Model file for the job. Use its own axes, mm. Face numbers are marked on the shaded views. A direction names the side the tool comes from. Round coordinates to 2 decimals unless told otherwise and drop trailing zeros. Order: outer loops, then holes, each group sorted by start corner. A loop starts at its lowest first (then second) coordinate and runs counter-clockwise, first axis right, second up. Notation, with made-up numbers: (48, 77.25) -> (83, 77.25) arc R22 cw to (83, 114.25) -> close; hole circle Ø11 at (-9.5, 26). An arc over 180 degrees is marked (long way). Answer as CSV lines item,"result".
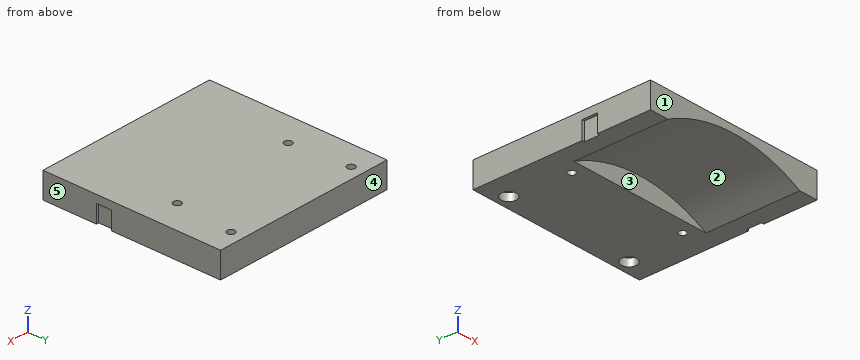
```python
from build123d import *

# Parameters (mm, degrees)
BOX241_W           = 6
BOX241_H           = 6
BOX241_DEPTH       = 64
BOX240_W           = 6
BOX240_H           = 6
BOX240_DEPTH       = 64
CYLINDER_R         = 60.2
CYLINDER_DEPTH     = 52
CYLINDER1233_R     = 1.5
CYLINDER1233_DEPTH = 32
CYLINDER1232_R     = 1.5
CYLINDER1232_DEPTH = 32
CYLINDER1239_R     = 1.5
CYLINDER1239_DEPTH = 100
CYLINDER1238_R     = 1.5
CYLINDER1238_DEPTH = 100
CYLINDER1245_R     = 3
CYLINDER1245_DEPTH = 3
CYLINDER1244_R     = 3
CYLINDER1244_DEPTH = 3
CYLINDER544_R      = 1.5
CYLINDER544_DEPTH  = 50
CYLINDER550_R      = 1.5
CYLINDER550_DEPTH  = 50
CYLINDER556_R      = 1.5
CYLINDER556_DEPTH  = 50
CYLINDER549_R      = 1.5
CYLINDER549_DEPTH  = 50
CYLINDER535_R      = 1.5
CYLINDER535_DEPTH  = 100
CYLINDER538_R      = 1.5
CYLINDER538_DEPTH  = 100
CYLINDER583_R      = 1.5
CYLINDER583_DEPTH  = 100
CYLINDER584_R      = 1.5
CYLINDER584_DEPTH  = 100
BOX142_W           = 72
BOX142_H           = 70
BOX142_DEPTH       = 10


with BuildPart() as krychle241:
    # Box241 → Box241 (new body)
    with BuildSketch(Plane(origin=(87, -3, -93), x_dir=(1, 0, 0), z_dir=(0, 0, 1))):
        with Locations((3, 3)):
            Rectangle(BOX241_W, BOX241_H)
    extrude(amount=BOX241_DEPTH)


with BuildPart() as compound653:
    # Box240 → Box240 (new body)
    with BuildSketch(Plane(origin=(11, -3, -93), x_dir=(1, 0, 0), z_dir=(0, 0, 1))):
        with Locations((3, 3)):
            Rectangle(BOX240_W, BOX240_H)
    extrude(amount=BOX240_DEPTH)

    # Compound653: union Krychle241
    add(krychle241.part)


with BuildPart() as compound653_1:
    # Compound653 placement: moved
    add(compound653.part.moved(Location((-52, 0, 36))))


with BuildPart() as obj1:
    # Cylinder → Cylinder (new body)
    with BuildSketch(Plane(origin=(0, 13, -53), x_dir=(1, 0, 0), z_dir=(0, -1, 0))):
        Circle(CYLINDER_R)
    extrude(amount=CYLINDER_DEPTH)


with BuildPart() as obj2:
    # Cylinder1233 → Cylinder1233 (new body)
    with BuildSketch(Plane(origin=(78, 41, -42), x_dir=(1, 0, 0), z_dir=(0, 0, 1))):
        Circle(CYLINDER1233_R)
    extrude(amount=CYLINDER1233_DEPTH)


with BuildPart() as compound620:
    # Cylinder1232 → Cylinder1232 (new body)
    with BuildSketch(Plane(origin=(26, 41, -42), x_dir=(1, 0, 0), z_dir=(0, 0, 1))):
        Circle(CYLINDER1232_R)
    extrude(amount=CYLINDER1232_DEPTH)

    # Compound620: union obj2
    add(obj2.part)


with BuildPart() as compound620_1:
    # Compound620 placement: moved
    add(compound620.part.moved(Location((-52, 0, 36))))


with BuildPart() as obj3:
    # Cylinder1239 → Cylinder1239 (new body)
    with BuildSketch(Plane(origin=(14, 0, -60), x_dir=(1, 0, 0), z_dir=(0, 0, 1))):
        Circle(CYLINDER1239_R)
    extrude(amount=CYLINDER1239_DEPTH)


with BuildPart() as compound630:
    # Cylinder1238 → Cylinder1238 (new body)
    with BuildSketch(Plane(origin=(90, 0, -60), x_dir=(1, 0, 0), z_dir=(0, 0, 1))):
        Circle(CYLINDER1238_R)
    extrude(amount=CYLINDER1238_DEPTH)

    # Compound625: union obj3
    add(obj3.part)


with BuildPart() as compound630_1:
    # Compound625 placement: moved
    add(compound630.part.moved(Location((-52, 0, 0))))

    # Compound630: union Compound620
    add(compound620_1.part)


with BuildPart() as obj4:
    # Cylinder1245 → Cylinder1245 (new body)
    with BuildSketch(Plane(origin=(78, 41, -42), x_dir=(1, 0, 0), z_dir=(0, 0, 1))):
        Circle(CYLINDER1245_R)
    extrude(amount=CYLINDER1245_DEPTH)


with BuildPart() as compound634:
    # Cylinder1244 → Cylinder1244 (new body)
    with BuildSketch(Plane(origin=(26, 41, -42), x_dir=(1, 0, 0), z_dir=(0, 0, 1))):
        Circle(CYLINDER1244_R)
    extrude(amount=CYLINDER1244_DEPTH)

    # Compound634: union obj4
    add(obj4.part)


with BuildPart() as compound634_1:
    # Compound634 placement: moved
    add(compound634.part.moved(Location((-52, 0, 42))))


with BuildPart() as obj5:
    # Cylinder544 → Cylinder544 (new body)
    with BuildSketch(Plane(origin=(-51, 6, 0), x_dir=(1, 0, 0), z_dir=(0, 0, 1))):
        Circle(CYLINDER544_R)
    extrude(amount=CYLINDER544_DEPTH)


with BuildPart() as obj6:
    # Cylinder550 → Cylinder550 (new body)
    with BuildSketch(Plane(origin=(-24, 18, 0), x_dir=(1, 0, 0), z_dir=(0, 0, 1))):
        Circle(CYLINDER550_R)
    extrude(amount=CYLINDER550_DEPTH)


with BuildPart() as obj7:
    # Cylinder556 → Cylinder556 (new body)
    with BuildSketch(Plane(origin=(24, 18, 0), x_dir=(1, 0, 0), z_dir=(0, 0, 1))):
        Circle(CYLINDER556_R)
    extrude(amount=CYLINDER556_DEPTH)


with BuildPart() as compound324:
    # Cylinder549 → Cylinder549 (new body)
    with BuildSketch(Plane(origin=(51, 6, 0), x_dir=(1, 0, 0), z_dir=(0, 0, 1))):
        Circle(CYLINDER549_R)
    extrude(amount=CYLINDER549_DEPTH)

    # Compound324: union obj5, obj6, obj7
    add(obj5.part)
    add(obj6.part)
    add(obj7.part)


with BuildPart() as obj8:
    # Cylinder535 → Cylinder535 (new body)
    with BuildSketch(Plane(origin=(51, -12, 0), x_dir=(1, 0, 0), z_dir=(0, 0, 1))):
        Circle(CYLINDER535_R)
    extrude(amount=CYLINDER535_DEPTH)


with BuildPart() as compound323:
    # Cylinder538 → Cylinder538 (new body)
    with BuildSketch(Plane(origin=(-51, -12, 0), x_dir=(1, 0, 0), z_dir=(0, 0, 1))):
        Circle(CYLINDER538_R)
    extrude(amount=CYLINDER538_DEPTH)

    # Compound323: union obj8
    add(obj8.part)


with BuildPart() as obj9:
    # Cylinder583 → Cylinder583 (new body)
    with BuildSketch(Plane(origin=(39, -21, 0), x_dir=(1, 0, 0), z_dir=(0, 0, 1))):
        Circle(CYLINDER583_R)
    extrude(amount=CYLINDER583_DEPTH)


with BuildPart() as compound628:
    # Cylinder584 → Cylinder584 (new body)
    with BuildSketch(Plane(origin=(-39, -21, 0), x_dir=(1, 0, 0), z_dir=(0, 0, 1))):
        Circle(CYLINDER584_R)
    extrude(amount=CYLINDER584_DEPTH)

    # Compound339: union obj9
    add(obj9.part)

    # Compound628: union Compound324, Compound323
    add(compound324.part)
    add(compound323.part)


with BuildPart() as compound628_1:
    # Compound628 placement: moved
    add(compound628.part.moved(Location((0, 0, -10))))


with BuildPart() as cut209:
    # Box142 → Box142 (new body)
    with BuildSketch(Plane(origin=(-36, -24, 0), x_dir=(1, 0, 0), z_dir=(0, 0, 1))):
        with Locations((36, 35)):
            Rectangle(BOX142_W, BOX142_H)
    extrude(amount=BOX142_DEPTH)

    # Cut201: cut Compound628
    add(compound628_1.part, mode=Mode.SUBTRACT)

    # Cut202: cut Compound634
    add(compound634_1.part, mode=Mode.SUBTRACT)

    # Cut203: cut Compound630
    add(compound630_1.part, mode=Mode.SUBTRACT)

    # Cut208: cut obj1
    add(obj1.part, mode=Mode.SUBTRACT)

    # Cut209: cut Compound653
    add(compound653_1.part, mode=Mode.SUBTRACT)


solid = cut209.part
```
Q1. Saw through at C-C (x = 4). Write the cut outline in (y, z), plus the area to 3 significant figures.
Checks:
outline,"(-24, 7.07) -> (13, 7.07) -> (13, 0) -> (46, 0) -> (46, 10) -> (-24, 10) -> close"
area,"439 mm²"
Q2. Flat gauge pins, fed straight in: pin 1 (0.8 mm diameter, centred on x = -35.5, y = 0.5, fed in from -Z); pin 2 (3 mm diameter, centred on y = -1, z = 4.5, fed in from -X); pin 3 (3 mm diameter, centred on x = -25, y = 40.5, fed in from -Z). Where does each tip first touch, or does it go through?
Checks:
pin 1,"z = 7"
pin 2,"x = -35"
pin 3,"z = 3"
Q3. Saw through at B-B (z = 5.25). Write the cut outline in (x, y).
Checks:
outline,"(-36, -24) -> (-15.2, -24) -> (-15.2, 13) -> (15.2, 13) -> (15.2, -24) -> (36, -24) -> (36, -3) -> (35, -3) -> (35, 3) -> (36, 3) -> (36, 46) -> (-36, 46) -> (-36, 3) -> (-35, 3) -> (-35, -3) -> (-36, -3) -> close; hole circle Ø3 at (-26, 41); hole circle Ø3 at (-24, 18); hole circle Ø3 at (24, 18); hole circle Ø3 at (26, 41)"
Q4. Wall check: L1, parallel to X at y = 18, z = 6; L2, parallel to X at y = 41, z = 5.75; L3, parallel to Y at x = 24, z = 5. Give the ranges that are in metal, low to high. Write a range as [from, to].
Checks:
L1,"[-36, -25.5], [-22.5, 22.5], [25.5, 36]"
L2,"[-36, -27.5], [-24.5, 24.5], [27.5, 36]"
L3,"[-24, 16.5], [19.5, 46]"
Q5. Saw through at A-A (y = 18). Write the cut outline in (x, z).
Checks:
outline,"(-36, 0) -> (-25.5, 0) -> (-25.5, 10) -> (-36, 10) -> close; (-22.5, 0) -> (22.5, 0) -> (22.5, 10) -> (-22.5, 10) -> close; (25.5, 0) -> (36, 0) -> (36, 10) -> (25.5, 10) -> close"
Q6. Tool access for the marked faces 1 and 2: list every direction of +Z, -Z, +X, -X, +Y, -Y with a clear straight run to the whole face (end or side of a thin tool).
Checks:
face 1,"+Z, -Z, +X, -X, -Y"
face 2,"-Z, -Y"
Q7. Mould opens along X. For the marked faces 3, 4 and 5 say: +X half, -X half, draft (parallel to the pull), parting line (faces both ways), or undercut.
Checks:
face 3,"undercut"
face 4,"draft"
face 5,"+X half"
